Verification items for the finished model (mm, model axes). A direction names the side the tool comes from. Round coordinates to 2 decimals unless told otherwise and drop trailing zeros. Loops run counter-clockwise (first coordinate to the right, second up) from the corner with the lowest first, then second, coordinate; pieces in that order, holes last.
from build123d import *

# Parameters (mm, degrees)
SKETCH1_R           = 2
BOSS_EXTRUDE1_DEPTH = 12
SKETCH4_W           = 35
SKETCH4_H           = 5
CUT_EXTRUDE1_DEPTH  = 113.433125829
FILLET2_R           = 10
FILLET3_R           = 1
CUT_EXTRUDE2_DEPTH  = 12


with BuildPart() as part:
    # Sketch1 → Boss-Extrude1 (new body)
    with BuildSketch(Plane(origin=(0, 0, 0), x_dir=(1, 0, 0), z_dir=(0, 1, 0))):
        with BuildLine():
            Line((100.816274371, -14.757411095), (17.5, 5))
            Line((17.5, 5), (-17.5, 5))
            Line((-17.5, 5), (-17.5, -5))
            Line((-17.5, -5), (17.5, -5))
            Line((17.5, -5), (29.181673037, -11.258392105))
            Line((29.181673037, -11.258392105), (30.466555694, -21.314125588))
            Line((30.466555694, -21.314125588), (31.091317661, -20.709888136))
            Line((31.091317661, -20.709888136), (31.94121893, -21.588658537))
            Line((31.94121893, -21.588658537), (32.591317661, -20.709888136))
            Line((32.591317661, -20.709888136), (33.316274371, -21.459469908))
            Line((33.316274371, -21.459469908), (34.091317661, -20.709888136))
            Line((34.091317661, -20.709888136), (34.816274371, -21.459469908))
            Line((34.816274371, -21.459469908), (35.591317661, -20.709888136))
            Line((35.591317661, -20.709888136), (36.316274371, -21.459469908))
            Line((36.316274371, -21.459469908), (37.091317661, -20.709888136))
            Line((37.091317661, -20.709888136), (37.816274371, -21.459469908))
            Line((37.816274371, -21.459469908), (38.591317661, -20.709888136))
            Line((38.591317661, -20.709888136), (39.316274371, -21.459469908))
            Line((39.316274371, -21.459469908), (40.091317661, -20.709888136))
            Line((40.091317661, -20.709888136), (40.816274371, -21.459469908))
            Line((40.816274371, -21.459469908), (41.591317661, -20.709888136))
            Line((41.591317661, -20.709888136), (42.316274371, -21.459469908))
            Line((42.316274371, -21.459469908), (43.091317661, -20.709888136))
            Line((43.091317661, -20.709888136), (43.816274371, -21.459469908))
            Line((43.816274371, -21.459469908), (44.591317661, -20.709888136))
            Line((44.591317661, -20.709888136), (45.316274371, -21.459469908))
            Line((45.316274371, -21.459469908), (46.091317661, -20.709888136))
            Line((46.091317661, -20.709888136), (46.816274371, -21.459469908))
            Line((46.816274371, -21.459469908), (47.591317661, -20.709888136))
            Line((47.591317661, -20.709888136), (48.316274371, -21.459469908))
            ThreePointArc((48.316274371, -21.459469908), (55.82900513, -18.797151194), (63.341735888, -21.459469908))
            Line((63.341735888, -21.459469908), (64.091317661, -20.709888136))
            Line((64.091317661, -20.709888136), (64.816274371, -21.459469908))
            Line((64.816274371, -21.459469908), (65.591317661, -20.709888136))
            Line((65.591317661, -20.709888136), (66.316274371, -21.459469908))
            Line((66.316274371, -21.459469908), (67.091317661, -20.709888136))
            Line((67.091317661, -20.709888136), (67.816274371, -21.459469908))
            Line((67.816274371, -21.459469908), (68.591317661, -20.709888136))
            Line((68.591317661, -20.709888136), (69.316274371, -21.459469908))
            Line((69.316274371, -21.459469908), (70.091317661, -20.709888136))
            Line((70.091317661, -20.709888136), (70.816274371, -21.459469908))
            Line((70.816274371, -21.459469908), (71.591317661, -20.709888136))
            Line((71.591317661, -20.709888136), (72.316274371, -21.459469908))
            Line((72.316274371, -21.459469908), (73.091317661, -20.709888136))
            Line((73.091317661, -20.709888136), (73.816274371, -21.459469908))
            Line((73.816274371, -21.459469908), (74.591317661, -20.709888136))
            Line((74.591317661, -20.709888136), (75.316274371, -21.459469908))
            Line((75.316274371, -21.459469908), (76.091317661, -20.709888136))
            Line((76.091317661, -20.709888136), (76.816274371, -21.459469908))
            Line((76.816274371, -21.459469908), (77.591317661, -20.709888136))
            Line((77.591317661, -20.709888136), (78.316274371, -21.459469908))
            Line((78.316274371, -21.459469908), (79.091317661, -20.709888136))
            Line((79.091317661, -20.709888136), (79.816274371, -21.459469908))
            Line((79.816274371, -21.459469908), (80.591317661, -20.709888136))
            Line((80.591317661, -20.709888136), (81.316274371, -21.459469908))
            Line((81.316274371, -21.459469908), (82.091317661, -20.709888136))
            Line((82.091317661, -20.709888136), (82.816274371, -21.459469908))
            Line((82.816274371, -21.459469908), (83.591317661, -20.709888136))
            Line((83.591317661, -20.709888136), (84.316274371, -21.459469908))
            Line((84.316274371, -21.459469908), (85.091317661, -20.709888136))
            Line((85.091317661, -20.709888136), (85.816274371, -21.459469908))
            Line((85.816274371, -21.459469908), (86.591317661, -20.709888136))
            Line((86.591317661, -20.709888136), (87.316274371, -21.459469908))
            Line((87.316274371, -21.459469908), (88.091317661, -20.709888136))
            Line((88.091317661, -20.709888136), (88.816274371, -21.459469908))
            Line((88.816274371, -21.459469908), (89.591317661, -20.709888136))
            Line((89.591317661, -20.709888136), (90.316274371, -21.459469908))
            Line((90.316274371, -21.459469908), (91.091317661, -20.709888136))
            Line((91.091317661, -20.709888136), (91.816274371, -21.459469908))
            Line((91.816274371, -21.459469908), (92.591317661, -20.709888136))
            Line((92.591317661, -20.709888136), (93.316274371, -21.459469908))
            Line((93.316274371, -21.459469908), (94.091317661, -20.709888136))
            Line((94.091317661, -20.709888136), (94.816274371, -21.459469908))
            Line((94.816274371, -21.459469908), (95.591317661, -20.709888136))
            Line((95.591317661, -20.709888136), (96.316274371, -21.459469908))
            Line((96.316274371, -21.459469908), (97.091317661, -20.709888136))
            Line((97.091317661, -20.709888136), (97.816274371, -21.459469908))
            Line((97.816274371, -21.459469908), (98.591317661, -20.709888136))
            Line((98.591317661, -20.709888136), (99.316274371, -21.459469908))
            Line((99.316274371, -21.459469908), (100.091317661, -20.709888136))
            Line((100.091317661, -20.709888136), (100.816274371, -21.459469908))
            Line((100.816274371, -21.459469908), (101.591317661, -20.709888136))
            Line((101.591317661, -20.709888136), (102.316274371, -21.459469908))
            Line((102.316274371, -21.459469908), (103.091317661, -20.709888136))
            Line((103.091317661, -20.709888136), (103.816274371, -21.459469908))
            Line((103.816274371, -21.459469908), (104.591317661, -20.709888136))
            Line((104.591317661, -20.709888136), (105.316274371, -21.459469908))
            Line((105.316274371, -21.459469908), (106.091317661, -20.709888136))
            Line((106.091317661, -20.709888136), (106.816274371, -21.459469908))
            Line((106.816274371, -21.459469908), (107.591317661, -20.709888136))
            Line((107.591317661, -20.709888136), (108.316274371, -21.459469908))
            Line((108.316274371, -21.459469908), (109.091317661, -20.709888136))
            Line((109.091317661, -20.709888136), (109.816274371, -21.459469908))
            Line((109.816274371, -21.459469908), (110.553264048, -21.459469908))
            Line((110.553264048, -21.459469908), (108.108025111, -17.888455122))
            Line((108.108025111, -17.888455122), (100.816274371, -14.757411095))
        make_face()
        with Locations(Location((11.21, 0, 0), (0, 0, 270))):
            Circle(SKETCH1_R, mode=Mode.SUBTRACT)
        with Locations(Location((-12.5, 0, 0), (0, 0, 270))):
            Circle(SKETCH1_R, mode=Mode.SUBTRACT)
    extrude(amount=BOSS_EXTRUDE1_DEPTH)

    # Sketch4 → Cut-Extrude1 (cut, through all)
    with BuildSketch(Plane.XY.offset(5)):
        with Locations((0, 6)):
            Rectangle(SKETCH4_W, SKETCH4_H)
    extrude(amount=-CUT_EXTRUDE1_DEPTH, mode=Mode.SUBTRACT)

    # Fillet2
    fillet2_edges = [part.edges().sort_by_distance(p)[0] for p in [
        (29.181673037, 6, 11.258392105),
    ]]
    fillet(fillet2_edges, radius=FILLET2_R)

    # Fillet3
    # the kernel refuses this fillet: 1 mm, written as the material it takes off along each edge
    with BuildSketch(Plane(origin=(100.816274371, -0.216477457, 14.757411095), x_dir=(-0.9730157961539994, 0, -0.23073851094864703), z_dir=(0, 1, 0))) as fillet3_piece_1:
        with BuildLine():
            CenterArc((FILLET3_R * 0.0865909827585, FILLET3_R), FILLET3_R, 260.102093181, 9.897906819)
            Line((-FILLET3_R * 0.0853021285033, FILLET3_R * 0.0148843934336), (-FILLET3_R * 0.0887399907286, -FILLET3_R * 0.00481791869774))
            Line((-FILLET3_R * 0.0887399907286, -FILLET3_R * 0.00481791869774), (-FILLET3_R * 0.00173181965517, -FILLET3_R * 0.02))
            Line((-FILLET3_R * 0.00173181965517, -FILLET3_R * 0.02), (FILLET3_R * 0.0865909827585, -FILLET3_R * 0.02))
            Line((FILLET3_R * 0.0865909827585, -FILLET3_R * 0.02), (FILLET3_R * 0.0865909827585, 0))
        make_face()
    extrude(amount=12.432954914, mode=Mode.SUBTRACT)
    with BuildSketch(Plane(origin=(108.108025111, -0.725377826, 17.888455122), x_dir=(-0.9188706856920634, 0, -0.3945588206792459), z_dir=(0, 1, 0))) as fillet3_piece_2:
        with BuildLine():
            CenterArc((FILLET3_R * 0.29015113035, FILLET3_R), FILLET3_R, 237.639707831, 32.360292169)
            Line((-FILLET3_R * 0.245090389396, FILLET3_R * 0.155300931965), (-FILLET3_R * 0.255795219791, FILLET3_R * 0.138406950604))
            Line((-FILLET3_R * 0.255795219791, FILLET3_R * 0.138406950604), (-FILLET3_R * 0.005803022607, -FILLET3_R * 0.02))
            Line((-FILLET3_R * 0.005803022607, -FILLET3_R * 0.02), (FILLET3_R * 0.29015113035, -FILLET3_R * 0.02))
            Line((FILLET3_R * 0.29015113035, -FILLET3_R * 0.02), (FILLET3_R * 0.29015113035, 0))
        make_face()
    extrude(amount=13.450755652, mode=Mode.SUBTRACT)
    with BuildSketch(Plane(origin=(110.553264048, -3.340980233, 21.459469908), x_dir=(-0.56498494903948, 0, -0.8251012103729192), z_dir=(0, 1, 0))) as fillet3_piece_3:
        with BuildLine():
            CenterArc((1.336392093, 1), FILLET3_R, 203.073330595, 66.926669405)
            Line((0.416388075, 0.608091074), (0.397987995, 0.600252896))
            ThreePointArc((0.397987995, 0.600252896), (0.191692013, 0.315345236), (-0.016502024, 0.011299699))
            Line((-0.016502024, 0.011299699), (0, -0.02))
            Line((0, -0.02), (1.336392093, -0.02))
            Line((1.336392093, -0.02), (1.336392093, 0))
        make_face()
    extrude(amount=18.681960466, mode=Mode.SUBTRACT)

    # Sketch5 → Cut-Extrude2 (cut)
    with BuildSketch(Plane(origin=(0, 12, 0), x_dir=(1, 0, 0), z_dir=(0, 1, 0))):
        Polygon((19.332052257, 2.4424245), (28.526818603, 0.242248117), (23.41536762, -4.087850301), (18.747614926, 0), align=None)
        Polygon((25.921082251, -6.661828657), (32.046043612, -11.428585655), (32.967525074, -16.9883699), (47.424517669, -16.9883699), (45.590433757, -4.934746753), (32.454936428, -1.421521761), align=None)
        Polygon((50.93529797, -7.151679552), (70.537795207, -11.282164386), (68.99785337, -18.590436131), align=None)
        Polygon((49.967342783, -8.662131451), (63.701149707, -17.359553871), (49.967342783, -17.061744713), align=None)
        Polygon((71.772087814, -18.590436131), (98.977842755, -18.590436131), (73.60079207, -11.778158935), align=None)
    extrude(amount=-CUT_EXTRUDE2_DEPTH, mode=Mode.SUBTRACT)


solid = part.part
1. Tool access check on faces 4 (the face through (104.417, 5.916, 16.304)), 5 (the face through (26, 6.1, 1.9)). Record the directions out of +Z, -Z, +X, -X, +Y, -Y that give a thin tool (end or side, any length) a straight path to the whole face; none if there is none.
2. Section check C-C (y = 6.5). Give the number of separate pieces and of enclosed holes in the cut face, then the cut area to 3 significant figures.
3. Section check D-D (x = 52). Enter the section's corners in (y, z).
4. Section check B-B (x = 11.21). Enter the section's corners in (y, z).
5. Release check for a two-part mould opening along X. For faces 1 (the face through (69.779, 6.084, 14.885)), 2 (the face through (36, 0, 2)), 3 (the face through (-17.5, 2, 0)) record: released by +X, released by -X, zero draft, split by the parting line, or undercut.
6. Scan lines: L1, parallel to Z at x = -12.5, y = 1.8; L2, parallel to Z at x = -5, y = 10.75; L3, parallel to Z at x = 75, y = 1.75. Record each from-to range of solid material in increasing order.
7. Section check A-A (x = -6.5). Enter the section's corners in (y, z), then the cut area to 3 significant figures.
8. Gauge pin test, flat ends, axial feed: P1, Ø5, axis at x = 3, y = 3.5, coming from the +Z side; P2, Ø4, axis at y = 6.5, z = 15.5, coming from the -X side; P3, Ø6, axis at x = 42, y = 5.5, coming from the -Z side. Record the tip position at first contact, or that the pin passes through.
Taken from the geometry:
1. face 4: -Z, +X, +Y, -Y
1. face 5: +Y, -Y
2. separate pieces: 1
2. enclosed holes: 5
2. area: 730 mm2
3. outline: (0, 3.18) - (12, 3.18) - (12, 7.38) - (0, 7.38) - close; (0, 7.83) - (12, 7.83) - (12, 9.95) - (0, 9.95) - close; (0, 17.11) - (12, 17.11) - (12, 19.43) - (0, 19.43) - close
4. outline: (0, -5) - (3.5, -5) - (3.5, -2) - (0, -2) - close; (0, 2) - (3.5, 2) - (3.5, 5) - (0, 5) - close; (8.5, -5) - (12, -5) - (12, -2) - (8.5, -2) - close; (8.5, 2) - (12, 2) - (12, 5) - (8.5, 5) - close
5. face 1: undercut
5. face 2: zero draft
5. face 3: released by -X
6. L1: z = -5 to -2, 2 to 5
6. L2: z = -5 to 5
6. L3: z = 8.64 to 12.15, 18.59 to 21.13
7. outline: (0, -5) - (3.5, -5) - (3.5, 5) - (0, 5) - close; (8.5, -5) - (12, -5) - (12, 5) - (8.5, 5) - close
7. area: 70.0 mm2
8. P1: stops at z = 5
8. P2: stops at x = 29.02
8. P3: stops at z = 0.1
